Could you check a few things on this model? Use its own coordinates, in mm. A direction names the side the tool comes from. Give positions to 0.01 mm unless a question says otherwise; leave off trailing zeros. Loops run counter-clockwise (first coordinate to the right, second up) from the corner with the lowest first, then second, coordinate; pieces in that order, holes last. Notation, with made-up numbers: M -14,24 L 10,24 A19 cw 10,35 Z; hole C 48,11 d7. An arc over 180 degrees is marked long. Answer in a Markdown table with one row per item. Add a question column.
```python
from build123d import *

# Parameters (mm, degrees)
EXTRUDE_1_DEPTH     = 13
SKETCH_2_W          = 19.25
SKETCH_2_H          = 7
CUT_EXTRUDE_1_DEPTH = 16
SKETCH_3_R          = 1.75
CUT_EXTRUDE_2_DEPTH = 6
FILLET_1_R          = 4
FILLET_2_R          = 1
FILLET_3_R          = 1
FILLET_4_R          = 0.5


with BuildPart() as part:
    # 草图1 → 凸台-拉伸1 (new, symmetric)
    with BuildSketch(Plane.XY):
        Polygon((0, -0.75), (17.75, -0.75), (17.75, -10.75), (27.25, -10.75), (27.25, -6), (25.75, -6), (25.75, -9.25), (19.25, -9.25), (19.25, 0.75), (0, 0.75), align=None)
    extrude(amount=EXTRUDE_1_DEPTH, both=True)

    # 草图2 → 切除-拉伸1 (cut)
    with BuildSketch(Plane(origin=(0, 0.75, 0), x_dir=(1, 0, 0), z_dir=(0, 1, 0))):
        with Locations((17.625, 9.5)):
            Rectangle(SKETCH_2_W, SKETCH_2_H)
        with Locations((17.625, -9.5)):
            Rectangle(SKETCH_2_W, SKETCH_2_H)
    extrude(amount=-CUT_EXTRUDE_1_DEPTH, mode=Mode.SUBTRACT)

    # 草图3 → 切除-拉伸2 (cut)
    with BuildSketch(Plane(origin=(0, 0.75, 0), x_dir=(1, 0, 0), z_dir=(0, 1, 0))):
        with Locations(Location((4, 8.25, 0), (0, 0, 270))):
            Circle(SKETCH_3_R)
        with Locations(Location((4, -8.25, 0), (0, 0, 270))):
            Circle(SKETCH_3_R)
    extrude(amount=-CUT_EXTRUDE_2_DEPTH, mode=Mode.SUBTRACT)

    # 圆角1
    fillet_1_edges = [part.edges().sort_by_distance(p)[0] for p in [
        (8, 0, 13),
        (0, 0, 13),
        (0, 0, -13),
        (8, 0, -13),
    ]]
    fillet(fillet_1_edges, radius=FILLET_1_R - 0.0001)  # a hair under: the kernel refuses the full size

    # 圆角2
    fillet_2_edges = [part.edges().sort_by_distance(p)[0] for p in [
        (8, 0, -6),
        (8, 0, 6),
    ]]
    fillet(fillet_2_edges, radius=FILLET_2_R)

    # 圆角3
    fillet_3_edges = [part.edges().sort_by_distance(p)[0] for p in [
        (19.25, 0.75, 0),
        (19.25, -9.25, 0),
        (25.75, -9.25, 0),
        (27.25, -10.75, 0),
        (17.75, -10.75, 0),
        (17.75, -0.75, 0),
    ]]
    fillet(fillet_3_edges, radius=FILLET_3_R)

    # 圆角4
    fillet_4_edges = [part.edges().sort_by_distance(p)[0] for p in [
        (25.75, -6, 0),
        (27.25, -6, 0),
    ]]
    fillet(fillet_4_edges, radius=FILLET_4_R)


solid = part.part
```
Item 1: Suppose I cut it at C-C (x = 21). List the corners of the cut face in (y, z) for me.
Item 2: If we mould it in two halves opening along X, with no side actions, what happens to faces 1 (the face through (19, -5, 6)), 2 (the face through (19.535, -8.949, 0.084)), 3 (the face through (1.141, -0.01, -11.797))? For each: +X half, -X half, draft (parallel to the pull), parting line (faces both ways), or undercut.
Item 3: For faces 4 (the face through (8, 0, 8)), 5 (the face through (8, 0, -8)), 6 (the face through (17.75, -6, 0)), which set-ups out of +Z, -Z, +X, -X, +Y, -Y let a thin tool reach every point of the face, with its end or its side?
Item 4: I need wall thicknesses on L1, parallel to X at y = 0.25, z = -8.25; L2, parallel to X at y = -8, z = -3.25; L3, parallel to Y at x = 12.25, z = 4.5. Which ranges of each line are inside material? Lowest first, please.
Item 5: Suppose I cut it at A-A (z = 8.25). List the corners of the cut face in (x, y) for me.
Item 6: Suppose I cut it at D-D (y = -3.25). List the corners of the cut face in (x, z) for me, then the cut area to 3 significant figures.
Item 7: For P1, Ø0.5, axis at y = -7, z = -2.5, coming from the -X side; P2, Ø12, axis at x = 7, z = -8, coming from the -Y side; P3, Ø1.3, axis at x = 21.5, z = -1, coming from the +Y side, each with a flat end and sliding along its axis, tell me the tip position at first contact or that it passes through.
Item 8: Suppose I cut it at B-B (z = -3.5). List the corners of the cut face in (x, y) for me.
Values found:
| question | item | result |
|---|---|---|
| 1 | outline | M -10.75,-6 L -9.25,-6 L -9.25,6 L -10.75,6 Z |
| 2 | face 1 | draft |
| 2 | face 2 | undercut |
| 2 | face 3 | -X half |
| 3 | face 4 | +Z, +X, +Y, -Y |
| 3 | face 5 | -Z, +X, +Y, -Y |
| 3 | face 6 | +Z, -Z, -X, -Y |
| 4 | L1 | 0 to 2.25, 5.75 to 8 |
| 4 | L2 | 17.75 to 19.25, 25.75 to 27.25 |
| 4 | L3 | -0.75 to 0.75 |
| 5 | outline | M 0,-0.75 L 2.25,-0.75 L 2.25,0.75 L 0,0.75 Z; M 5.75,-0.75 L 8,-0.75 L 8,0.75 L 5.75,0.75 Z |
| 6 | outline | M 17.75,-6 L 19.25,-6 L 19.25,6 L 17.75,6 Z |
| 6 | area | 18.0 mm² |
| 7 | P1 | x = 17.75 |
| 7 | P2 | y = -0.75 |
| 7 | P3 | y = -9.25 |
| 8 | outline | M 0,-0.75 L 16.75,-0.75 A1 cw 17.75,-1.75 L 17.75,-9.75 A1 ccw 18.75,-10.75 L 26.25,-10.75 A1 ccw 27.25,-9.75 L 27.25,-6.5 A0.5 ccw 26.75,-6 L 26.25,-6 A0.5 ccw 25.75,-6.5 L 25.75,-8.25 A1 cw 24.75,-9.25 L 20.25,-9.25 A1 cw 19.25,-8.25 L 19.25,-0.25 A1 ccw 18.25,0.75 L 0,0.75 Z |
